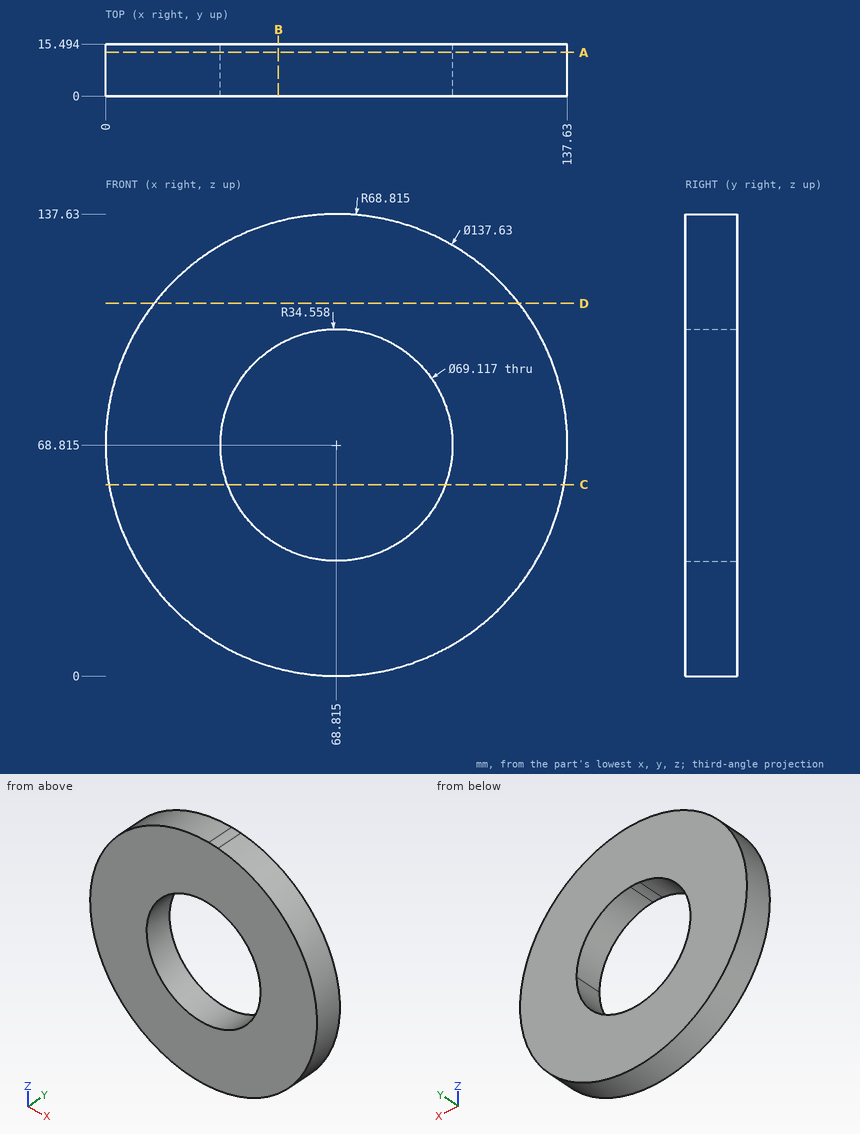
Part print with two shaded views. Sizes in mm from the minimum x, y, z corner. Round coordinates to 2 decimals unless told otherwise and drop trailing zeros. Write each loop counter-clockwise with the first axis right and the second up, starting at its lowest first coordinate (ties: lowest second). Pieces come first, ordered by that corner, then holes. Notation, with made-up numbers: M 88.5,-8.75 L 143.5,-8.75 A34 ccw 143.5,28.25 Z; hole C -32.75,49 d10. An arc over 180 degrees is marked long. Put each result on its own line as item: value. Start each with the question number.
1) Saw through at D-D, the plane z = 111. Write the cut outline in (x, y), and give its area (4 significant figures).
2) Saw through at B-B, the plane x = 51.5. Write the cut outline in (y, z).
3) Saw through at A-A, the plane y = 13. Write the cut outline in (x, z) (1 decimal).
4) Saw through at C-C, the plane z = 57. Write the cut outline in (x, y), and give its area (3 significant figures).
5) Pin check, flat tips, straight feed: pin 1 Ø6 at (x, y) = (74, 10.5) entering from +Z (1 decimal); pin 2 Ø5 at (x, y) = (122.5, 13.5) entering from -Z; pin 3 Ø1.5 at (y, z) = (10.5, 92.5) entering from +X (1 decimal). Stop position of each tip, or through.
6) Drill centre lines: probe 1 along Z at (x, y) = (98, 10) (1 decimal); probe 2 along Z at (x, y) = (43.5, 4.25) (1 decimal); probe 3 along X at (y, z) = (1.5, 99.5) (1 decimal). Where is each one in solid material? Low to high. Write a range as [from, to].
Resolved:
1. outline: M 14.45,0 L 123.18,0 L 123.18,15.49 L 14.45,15.49 Z
1. area: 1,685 mm²
2. outline: M 0,2.21 L 15.49,2.21 L 15.49,38.91 L 0,38.91 Z; M 0,98.72 L 15.49,98.72 L 15.49,135.42 L 0,135.42 Z
3. outline: C 68.8,68.8 d137.6; hole C 68.8,68.8 d69.1
4. outline: M 1.02,0 L 36.34,0 L 36.34,15.49 L 1.02,15.49 Z; M 101.29,0 L 136.61,0 L 136.61,15.49 L 101.29,15.49 Z
4. area: 1,090 mm²
5. pin 1: z = 137.6
5. pin 2: z = 22.82
5. pin 3: x = 133.7
6. probe 1: [6.5, 50.3], [87.3, 131.1]
6. probe 2: [4.8, 45.3], [92.3, 132.8]
6. probe 3: [7.2, 52.9], [84.7, 130.4]
